```python
from build123d import *

# Parameters (mm, degrees)
F1_DEPTH = 25.4


with BuildPart() as f1:
    # F0 (on Top) → F1 (new body)
    with BuildSketch(Plane.XY):
        with BuildLine():
            ThreePointArc((44.45, 41.275), (43.520064, 43.520064), (41.275, 44.45))
            Line((41.275, 44.45), (-15.120606, 44.45))
            Line((-15.120606, 44.45), (-44.45, -6.35))
            Line((-44.45, -6.35), (-44.45, -41.275))
            ThreePointArc((-44.45, -41.275), (-43.520064, -43.520064), (-41.275, -44.45))
            Line((-41.275, -44.45), (41.275, -44.45))
            ThreePointArc((41.275, -44.45), (43.520064, -43.520064), (44.45, -41.275))
            Line((44.45, -41.275), (44.45, 41.275))
        make_face()
    extrude(amount=F1_DEPTH)


solid = f1.part
```
Geometry check sheet. Reference: the model listing, model coordinates, mm. Give positions to 0.01 mm unless a question says otherwise; leave off trailing zeros. Write each loop counter-clockwise with the first axis right and the second up, starting at its lowest first coordinate (ties: lowest second). Pieces come first, ordered by that corner, then holes.
1) Release check for a two-part mould opening along X. For faces 1 (the cylindrical face through (43.5, -43.54, 12.52)), 2 (the flat face through (-44.45, -24, 13)), 3 (the flat face through (-1, 1, 0)) record: pulls with the +X half, pulls with the -X half, needs draft (parallel to the pull), parting line crosses it, or undercut.
2) Material ranges on L1, parallel to X at y = 36.5, z = 3.75; L2, parallel to X at y = -6, z = 5; L3, parallel to Y at x = -37, z = 13.5, recorded low to high.
3) Section check A-A, the plane z = 23. Record the boundary of the cut face in (x, y) (3 decimals).
4) Section check B-B, the plane y = 34.5. Record the boundary of the cut face in (x, z), and give its area (3 significant figures).
5) Section check C-C, the plane y = 21. Record the boundary of the cut face in (x, z), and give its area (3 significant figures).
6) Gauge pin test, flat end, axial feed: pin 1 (8 mm diameter, centred on y = 7, z = 9.5, fed in from -X). Record the tip position at first contact, or that the pin passes through.
Computed:
1. face 1: pulls with the +X half
1. face 2: pulls with the -X half
1. face 3: needs draft
2. L1: x = -19.71 to 44.45
2. L2: x = -44.25 to 44.45
2. L3: y = -44.45 to 6.55
3. outline: (-44.45, -41.275) arc R3.175 ccw to (-41.275, -44.45) - (41.275, -44.45) arc R3.175 ccw to (44.45, -41.275) - (44.45, 41.275) arc R3.175 ccw to (41.275, 44.45) - (-15.121, 44.45) - (-44.45, -6.35) - close
4. outline: (-20.87, 0) - (44.45, 0) - (44.45, 25.4) - (-20.87, 25.4) - close
4. area: 1,660 mm2
5. outline: (-28.66, 0) - (44.45, 0) - (44.45, 25.4) - (-28.66, 25.4) - close
5. area: 1,860 mm2
6. pin 1: stops at x = -39.05
